from build123d import *

# Parameters (mm, degrees)
BOSS_EXTRUDE1_DEPTH = 25.4
SKETCH2_R           = 7.0739
SKETCH2_R_2         = 3.2639
BOSS_EXTRUDE2_DEPTH = 3.175
BOSS_EXTRUDE3_DEPTH = 3.302


with BuildPart() as part:
    # Sketch1 → Boss-Extrude1 (new body)
    with BuildSketch(Plane.XY):
        with BuildLine():
            ThreePointArc((70.001721328, 21.116929737), (32.109818913, 121.760822938), (121.667937999, 181.295122405))
            Line((121.667937999, 181.295122405), (282.867264941, 167.491822308))
            ThreePointArc((282.867264941, 167.491822308), (319.66332332, 132.52036188), (293.637822612, 88.935659637))
            Line((293.637822612, 88.935659637), (294.839214659, 85.723778364))
            Line((294.839214659, 85.723778364), (299.063190222, 87.84501085))
            ThreePointArc((299.063190222, 87.84501085), (322.426612475, 135.274348553), (283.138145015, 170.655245926))
            Line((283.138145015, 170.655245926), (121.938818073, 184.458546023))
            ThreePointArc((121.938818073, 184.458546023), (29.088121079, 122.735485546), (68.373108141, 18.391449213))
            Line((68.373108141, 18.391449213), (70.001721328, 21.116929737))
        make_face()
    extrude(amount=BOSS_EXTRUDE1_DEPTH)

    # Sketch2 → Boss-Extrude2 (add)
    # profile 1 of 2: a face of its own
    with BuildSketch(Plane(origin=(0, 0, 0), x_dir=(-1, 0, 0), z_dir=(0, 0, -1))):
        with BuildLine():
            ThreePointArc((-36.587701927, 50.782990283), (-44.384911147, 39.317928918), (-53.858754358, 29.194174745))
            Line((-53.858754358, 29.194174745), (-22.316186857, 12.775282108))
            ThreePointArc((-22.316186857, 12.775282108), (-23.932636358, 13.931413925), (-25.163710326, 15.491544259))
            ThreePointArc((-25.163710326, 15.491544259), (-23.930769686, 24.17036605), (-15.202863294, 24.986295173))
            ThreePointArc((-15.202863294, 24.986295173), (-14.373460165, 24.357545231), (-13.645291854, 23.613900861))
            Line((-13.645291854, 23.613900861), (-36.587701927, 50.782990283))
        make_face()
    # profile 2 of 2: a face of its own
    with BuildSketch(Plane(origin=(0, 0, 0), x_dir=(-1, 0, 0), z_dir=(0, 0, -1))):
        with Locations((-19.05, 19.05)):
            Circle(SKETCH2_R)
        with Locations((-19.05, 19.05)):
            Circle(SKETCH2_R_2, mode=Mode.SUBTRACT)
    extrude(amount=-BOSS_EXTRUDE2_DEPTH)

    # Sketch3 → Boss-Extrude3 (add)
    with BuildSketch(Plane.XY.offset(25.4)):
        with BuildLine():
            Line((68.373108141, 18.391449213), (70.001721328, 21.116929737))
            ThreePointArc((70.001721328, 21.116929737), (32.109818913, 121.760822938), (121.667937999, 181.295122405))
            Line((121.667937999, 181.295122405), (282.867264941, 167.491822308))
            ThreePointArc((282.867264941, 167.491822308), (319.66332332, 132.52036188), (293.637822612, 88.935659637))
            Line((293.637822612, 88.935659637), (294.839214659, 85.723778364))
            Line((294.839214659, 85.723778364), (299.063190222, 87.84501085))
            ThreePointArc((299.063190222, 87.84501085), (322.426612475, 135.274348553), (283.138145015, 170.655245926))
            Line((283.138145015, 170.655245926), (121.938818073, 184.458546023))
            ThreePointArc((121.938818073, 184.458546023), (29.088121079, 122.735485546), (68.373108141, 18.391449213))
        make_face()
    extrude(amount=BOSS_EXTRUDE3_DEPTH)


solid = part.part
Source: CAD feature listing. Evaluate the final solid. Frame: model axes, mm. A direction names the side the tool comes from. Coordinates: 2 decimals unless noted, no trailing zeros. Write each loop counter-clockwise with the first axis right and the second up, starting at its lowest first coordinate (ties: lowest second). Pieces come first, ordered by that corner, then holes. Notation, with made-up numbers: M -10.5,2.5 L 0.5,2.5 A31 cw 0.5,26.5 Z; hole C -3,44.5 d4. An arc over 180 degrees is marked long. Use a Markdown table: item, result.
1) Section C-C, the plane y = 102.5. Output: boundary loops of the cut face in (x, z).
Conclusion:
| item | result |
|---|---|
| outline | M 25.06,0 L 28.24,0 L 28.24,28.7 L 25.06,28.7 Z; M 311.82,0 L 315.72,0 L 315.72,28.7 L 311.82,28.7 Z |
2) Section A-A, the plane x = 19.05. Output: boundary loops of the cut face in (y, z) (3 decimals).
Conclusion:
| item | result |
|---|---|
| outline | M 11.976,0 L 15.786,0 L 15.786,3.175 L 11.976,3.175 Z; M 22.314,0 L 30.014,0 L 30.014,3.175 L 22.314,3.175 Z |
3) Ray query, L1, parallel to X at y = 148.5, z = 24.25; L2, parallel to Y at x = 19.05, z = 1.1; L3, parallel to X at y = 100, z = 25. Return the intervals inside material, ascending.
Conclusion:
| item | result |
|---|---|
| L1 | x = 42.32 to 46.31, 313.89 to 317.58 |
| L2 | y = 11.98 to 15.79, 22.31 to 30.01 |
| L3 | x = 24.89 to 28.07, 309.77 to 313.91 |
4) Section B-B, the plane z = 7.75. Output: boundary loops of the cut face in (x, y) (3 decimals), then the cut area to 3 significant figures.
Conclusion:
| item | result |
|---|---|
| outline | M 68.373,18.391 L 70.002,21.117 A86.36 cw 121.668,181.295 L 282.867,167.492 A40.64 cw 293.638,88.936 L 294.839,85.724 L 299.063,87.845 A43.815 ccw 283.138,170.655 L 121.939,184.459 A89.535 ccw Z |
| area | 1,630 mm^2 |
5) Section D-D, the plane y = 77.5. Output: boundary loops of the cut face in (x, z), then the cut area to 3 significant figures.
Conclusion:
| item | result |
|---|---|
| outline | M 26.54,0 L 29.78,0 L 29.78,28.7 L 26.54,28.7 Z |
| area | 93.0 mm^2 |
6) Reachability of faces 4 (the flat face through (33, 27, 3.175)), 5 (the cylindrical face through (319.55, 133.28, 14.15)), 6 (the flat face through (201.14, 174.49, 14.15)) from +Z, -Z, +X, -X, +Y, -Y: full face, straight path, thin tool, end or side. Return the list, or none.
Conclusion:
| item | result |
|---|---|
| face 4 | +Z, -X, -Y |
| face 5 | +Z, -Z |
| face 6 | +Z, -Z, -Y |
7) First-contact query: pin 1 Ø6 at (y, z) = (83, 24) entering from -X; pin 2 Ø1.5 at (y, z) = (132.5, 16.5) entering from +X; pin 3 Ø5 at (x, z) = (241, 21.5) entering from +Y. Flat tips, straight axial feed; report the tip coordinate or a pass-through.
Conclusion:
| item | result |
|---|---|
| pin 1 | stops at x = 25.24 |
| pin 2 | stops at x = 322.96 |
| pin 3 | stops at y = 174.48 |
8) Mould query, pull axis X, two halves, no side actions, for faces 1 (the cylindrical face through (22.31, 19.19, 1.57)), 2 (the cylindrical face through (13.61, 14.53, 1.57)), 3 (the flat face through (53, 156.4, 0)). Classes: pulls with the +X half, pulls with the -X half, needs draft (parallel to the pull), parting line crosses it, or undercut.
Conclusion:
| item | result |
|---|---|
| face 1 | undercut |
| face 2 | parting line crosses it |
| face 3 | needs draft |
